Build history of the part. All positions in model axes, mm. A direction names the side the tool comes from. Round coordinates to 2 decimals unless told otherwise and drop trailing zeros. Write each loop counter-clockwise with the first axis right and the second up, starting at its lowest first coordinate (ties: lowest second). Pieces come first, ordered by that corner, then holes. Notation, with made-up numbers: M -38,26.25 L -11,26.25 A29 cw -11,65.25 Z; hole C -12.75,-11 d3. An arc over 180 degrees is marked long. Use a Markdown table: item, result.
from build123d import *

# Parameters (mm, degrees)
SKETCH1_R           = 2.91
BOSS_EXTRUDE1_DEPTH = 15.53
CUT_EXTRUDE2_START  = -7.89
SKETCH2_R           = 2.91
SKETCH2_R_2         = 2.435
CUT_EXTRUDE2_DEPTH  = 7.89
SKETCH4_R           = 1.96
CUT_EXTRUDE3_DEPTH  = 7.89
CUT_EXTRUDE6_DEPTH  = 7.89
SKETCH10_R          = 2.91
SKETCH10_R_2        = 2.44
CUT_EXTRUDE10_DEPTH = 6.72


with BuildPart() as part:
    # Sketch1 → Boss-Extrude1 (new body)
    with BuildSketch(Plane.XY):
        Circle(SKETCH1_R)
    extrude(amount=BOSS_EXTRUDE1_DEPTH)

    # Sketch2 → Cut-Extrude2 (cut)
    with BuildSketch(Plane.XY.offset(15.53).offset(CUT_EXTRUDE2_START)):
        Circle(SKETCH2_R)
        Circle(SKETCH2_R_2, mode=Mode.SUBTRACT)
    extrude(amount=CUT_EXTRUDE2_DEPTH, mode=Mode.SUBTRACT)

    # Sketch4 → Cut-Extrude3 (cut)
    with BuildSketch(Plane.XY.offset(15.53)):
        Circle(SKETCH4_R)
    extrude(amount=-CUT_EXTRUDE3_DEPTH, mode=Mode.SUBTRACT)

    # Sketch6 → Cut-Extrude6 (cut)
    with BuildSketch(Plane(origin=(-2.06167752, -1.295650727, 0), x_dir=(0, 0, 1), z_dir=(-0.8466848129866222, -0.5320947542100077, 0))):
        with BuildLine():
            Line((15.53, -0.5), (13.28, -0.5))
            ThreePointArc((13.28, -0.5), (12.78, 0), (13.28, 0.5))
            Line((13.28, 0.5), (15.53, 0.5))
            ThreePointArc((15.53, 0.5), (16.03, 0), (15.53, -0.5))
        make_face()
    extrude(amount=-CUT_EXTRUDE6_DEPTH, mode=Mode.SUBTRACT)

    # Sketch10 → Cut-Extrude10 (cut)
    # profile 1 of 5: a face of its own
    with BuildSketch(Plane(origin=(0, 0, 0), x_dir=(-1, 0, 0), z_dir=(0, 0, -1))):
        Circle(SKETCH10_R)
        Circle(SKETCH10_R_2, mode=Mode.SUBTRACT)
    # profile 2 of 5: a face of its own
    with BuildSketch(Plane(origin=(0, 0, 0), x_dir=(-1, 0, 0), z_dir=(0, 0, -1))):
        with BuildLine():
            Line((-2.273845861, 0.885), (-0.885, 0.885))
            Line((-0.885, 0.885), (-0.885, 2.273845861))
            ThreePointArc((-0.885, 2.273845861), (-1.725340546, 1.725340546), (-2.273845861, 0.885))
        make_face()
    # profile 3 of 5: a face of its own
    with BuildSketch(Plane(origin=(0, 0, 0), x_dir=(-1, 0, 0), z_dir=(0, 0, -1))):
        with BuildLine():
            Line((0.885, 2.273845861), (0.885, 0.885))
            Line((0.885, 0.885), (2.273845861, 0.885))
            ThreePointArc((2.273845861, 0.885), (1.725340546, 1.725340546), (0.885, 2.273845861))
        make_face()
    # profile 4 of 5: a face of its own
    with BuildSketch(Plane(origin=(0, 0, 0), x_dir=(-1, 0, 0), z_dir=(0, 0, -1))):
        with BuildLine():
            Line((0.885, -0.885), (0.885, -2.273845861))
            ThreePointArc((0.885, -2.273845861), (1.725340546, -1.725340546), (2.273845861, -0.885))
            Line((2.273845861, -0.885), (0.885, -0.885))
        make_face()
    # profile 5 of 5: a face of its own
    with BuildSketch(Plane(origin=(0, 0, 0), x_dir=(-1, 0, 0), z_dir=(0, 0, -1))):
        with BuildLine():
            ThreePointArc((-2.273845861, -0.885), (-1.725340546, -1.725340546), (-0.885, -2.273845861))
            Line((-0.885, -2.273845861), (-0.885, -0.885))
            Line((-0.885, -0.885), (-2.273845861, -0.885))
        make_face()
    extrude(amount=-CUT_EXTRUDE10_DEPTH, mode=Mode.SUBTRACT)


solid = part.part
Q1. Cut at A-A on z = 13.5. Give the cut face in (x, y) (3 decimals).
Response values:
| item | result |
|---|---|
| outline | M -2.284,-0.845 L -1.871,-0.585 A1.96 cw 1.339,1.432 L 1.752,1.691 A2.435 ccw Z; M -1.752,-1.691 A2.435 ccw 2.284,0.845 L 1.871,0.585 A1.96 cw -1.339,-1.432 Z |
Q2. Cut at B-B on y = 0. Give the cut face in (x, z) (3 decimals), and give its area (3 significant figures).
Response values:
| item | result |
|---|---|
| outline | M -2.91,6.72 L -2.44,6.72 L -2.44,0 L 2.44,0 L 2.44,6.72 L 2.91,6.72 L 2.91,7.64 L 2.435,7.64 L 2.435,15.53 L 1.96,15.53 L 1.96,7.64 L -1.96,7.64 L -1.96,15.53 L -2.435,15.53 L -2.435,7.64 L -2.91,7.64 Z |
| area | 45.6 mm2 |
Q3. Cut at D-D on z = 1. Give the cut face in (x, y) (3 decimals), and give its area (3 significant figures).
Response values:
| item | result |
|---|---|
| outline | M -2.274,-0.885 L -0.885,-0.885 L -0.885,-2.274 A2.44 ccw 0.885,-2.274 L 0.885,-0.885 L 2.274,-0.885 A2.44 ccw 2.274,0.885 L 0.885,0.885 L 0.885,2.274 A2.44 ccw -0.885,2.274 L -0.885,0.885 L -2.274,0.885 A2.44 ccw Z |
| area | 13.8 mm2 |
Q4. Drill centre lines: L1, parallel to Y at x = 0, z = 9.75 (3 decimals); L2, parallel to X at y = -2.1, z = 1.5 (3 decimals). Where is each one in solid material? Low to high.
Response values:
| item | result |
|---|---|
| L1 | y = -2.435 to -1.96, 1.96 to 2.435 |
| L2 | x = -0.885 to 0.885 |
Q5. Cut at C-C on x = 0.5. Give the cut face in (y, z).
Response values:
| item | result |
|---|---|
| outline | M -2.87,6.72 L -2.39,6.72 L -2.39,0 L 2.39,0 L 2.39,6.72 L 2.87,6.72 L 2.87,7.64 L 2.38,7.64 L 2.38,15.53 L 1.9,15.53 L 1.9,7.64 L -1.9,7.64 L -1.9,15.53 L -2.38,15.53 L -2.38,7.64 L -2.87,7.64 Z |
Q6. Which spindle directions (+Z, -Z, +X, -X, +Y, -Y) get a long thin tool onto all of the face, cutting with end or side? Do faces 4 (the flat face through (0.885, 2, 3)), 5 (the cylindrical face through (2.323, 0.731, 11.53)), 6 (the flat face through (-2, 0.885, 3)), 7 (the cylindrical face through (-2.44, -0.01, 3.31)). Say none if no direction does.
Response values:
| item | result |
|---|---|
| face 4 | -Z, +X, +Y |
| face 5 | +Z |
| face 6 | -Z, -X, +Y |
| face 7 | -Z, -X |
Q7. Drop flat-ended pins along their axis: P1, Ø1, axis at x = 1, z = 6, coming from the +Y side; P2, Ø1.1, axis at y = -1, z = 2, coming from the +X side; P3, Ø1.5, axis at x = -1.5, z = 3, coming from the +Y side. Give the stop position or say it passes through.
Response values:
| item | result |
|---|---|
| P1 | stops at y = 2.39 |
| P2 | stops at x = 2.4 |
| P3 | stops at y = 2.32 |
Q8. Two-plate mould, pull along Y, no slides. Class faces 1 (the cylindrical face through (-0.01, 2.44, 3.31)), 2 (the cylindrical face through (-1.83, -1.16, 12.78)), 3 (the flat face through (1, -2, 15.53)): +Y half, -Y half, draft (parallel to the pull), parting line (faces both ways), or undercut.
Response values:
| item | result |
|---|---|
| face 1 | +Y half |
| face 2 | undercut |
| face 3 | draft |
